```python
from build123d import *

# Parameters (mm, degrees)
SKETCH1_W                = 34
SKETCH1_H                = 24
BOSS_EXTRUDE1_DEPTH      = 10
SKETCH2_W                = 30
SKETCH2_H                = 20
CUT_EXTRUDE1_DEPTH       = 8
SKETCH3_W                = 16
SKETCH3_H                = 2
BOSS_EXTRUDE2_DEPTH      = 0.5
CHAMFER1_SIZE            = 0.5
SKETCH4_W                = 7
SKETCH4_H                = 7
BOSS_EXTRUDE3_DEPTH      = 3
FILLET1_R                = 3.5
SKETCH6_R                = 1.75
CUT_EXTRUDE2_DEPTH       = 29.635642127
CIRPATTERN2_COUNT        = 2
FILLET1_OF_CIRPATTERN2_R = 3.5
FILLET2_R                = 3.5


with BuildPart() as part:
    # Sketch1 → Boss-Extrude1 (new body)
    with BuildSketch(Plane.XY):
        Rectangle(SKETCH1_W, SKETCH1_H)
    extrude(amount=BOSS_EXTRUDE1_DEPTH)

    # Sketch2 → Cut-Extrude1 (cut)
    with BuildSketch(Plane.XY.offset(10)):
        Rectangle(SKETCH2_W, SKETCH2_H)
    extrude(amount=-CUT_EXTRUDE1_DEPTH, mode=Mode.SUBTRACT)

    # Sketch3 → Boss-Extrude2 (add)
    with BuildSketch(Plane.XZ.offset(-10)):
        with Locations((0, 9)):
            Rectangle(SKETCH3_W, SKETCH3_H)
    boss_extrude2 = extrude(amount=BOSS_EXTRUDE2_DEPTH)

    # Mirror1: Boss-Extrude2 across plane
    add(boss_extrude2.mirror(Plane.ZX))

    # Chamfer1
    chamfer1_edges = [part.edges().sort_by_distance(p)[0] for p in [
        (8, 10, 9),
        (-8, 10, 9),
        (-8, -10, 9),
        (8, -10, 9),
    ]]
    chamfer(chamfer1_edges, length=CHAMFER1_SIZE - 0.0001)  # a hair under: the kernel refuses the full size

    # Sketch4 → Boss-Extrude3 (add)
    with BuildSketch(Plane.XY):
        with Locations((20.5, 8.5)):
            Rectangle(SKETCH4_W, SKETCH4_H)
    boss_extrude3 = extrude(amount=BOSS_EXTRUDE3_DEPTH)

    # Fillet1
    fillet1_edges = [part.edges().sort_by_distance(p)[0] for p in [
        (24, 12, 1.5),
        (24, 5, 1.5),
    ]]
    fillet(fillet1_edges, radius=FILLET1_R - 0.0001)  # a hair under: the kernel refuses the full size

    # Sketch6 → Cut-Extrude2 (cut, through all)
    with BuildSketch(Plane(origin=(0, 0, 0), x_dir=(-1, 0, 0), z_dir=(0, 0, -1))):
        with Locations((-20.5, 8.5)):
            Circle(SKETCH6_R)
    cut_extrude2 = extrude(amount=-CUT_EXTRUDE2_DEPTH, mode=Mode.SUBTRACT)

    # CirPattern2: Boss-Extrude3, Cut-Extrude2 ×2 about axis
    cirpattern2_axis = Axis((0, 0, 0), (0, 0, 1))
    add([boss_extrude3.rotate(cirpattern2_axis, i * 360 / CIRPATTERN2_COUNT) for i in range(1, CIRPATTERN2_COUNT)])
    add([cut_extrude2.rotate(cirpattern2_axis, i * 360 / CIRPATTERN2_COUNT) for i in range(1, CIRPATTERN2_COUNT)], mode=Mode.SUBTRACT)

    # Fillet1 of CirPattern2
    fillet1_of_cirpattern2_edges = [part.edges().sort_by_distance(p)[0] for p in [
        (-24, -12, 1.5),
        (-24, -5, 1.5),
    ]]
    fillet(fillet1_of_cirpattern2_edges, radius=FILLET1_OF_CIRPATTERN2_R - 0.0001)  # a hair under: the kernel refuses the full size

    # Fillet2
    fillet2_edges = [part.edges().sort_by_distance(p)[0] for p in [
        (-17, -5, 1.5),
        (17, 5, 1.5),
    ]]
    fillet(fillet2_edges, radius=FILLET2_R)


solid = part.part
```
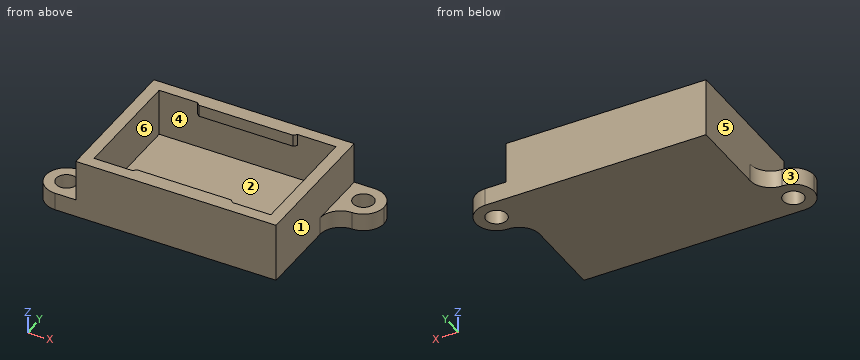
Design review of the part built by this model. Coordinates are the model's own, in mm. Face numbers are marked on the shaded views. A direction names the side the tool comes from. Round coordinates to 2 decimals unless told otherwise and drop trailing zeros. Order: outer loops, then holes, each group sorted by start corner. A loop starts at its lowest first (then second) coordinate and runs counter-clockwise, first axis right, second up. Notation, with made-up numbers: M 16.25,16 L 42.25,16 A15 cw 42.25,42 Z; hole C 23,-35.5 d11. An arc over 180 degrees is marked long. Put each result on its own line as item: value.
Q1. Insertion check: pin 1 Ø5 at (y, z) = (-3.5, 8.5) entering from +X; pin 2 Ø1 at (x, y) = (-3.5, 8.5) entering from +Z; pin 3 Ø3 at (y, z) = (3, 7) entering from -X. Each pin has a flat end and moves straight along its axis. Give the tip position at first contact, or say it passes through.
Reported:
pin 1: x = 17
pin 2: z = 2
pin 3: x = -17
Q2. Draft analysis for pull direction Y (two halves, no side actions). For the marked faces 1, 2 and 3, state which applies: released by +Y, released by -Y, zero draft, split by the parting line, or undercut.
Reported:
face 1: zero draft
face 2: undercut
face 3: released by +Y
Q3. Consider section B-B (z = 6). State the section outline as (x, y) points, and give its area (3 significant figures).
Reported:
outline: M -17,-12 L 17,-12 L 17,12 L -17,12 Z; hole M -15,-10 L 15,-10 L 15,10 L -15,10 Z
area: 216 mm²
Q4. Machinability: for the marked faces 4, 5 and 6, which of the approach directions +Z, -Z, +X, -X, +Y, -Y give a long, thin tool a straight path to every point of the face, cutting with its end or side? Answer none if there is none.
Reported:
face 4: none
face 5: +Z, -X, +Y
face 6: +Z
Q5. To check wall thickness, follow line 1 (Y direction, x = -20.5, z = 1.35); line 2 (Y direction, x = -4, z = 4.75); line 3 (X direction, y = -1.25, z = 3.5). State the ranges of each line that lie inside material, in increasing order.
Reported:
line 1: -12 to -10.25, -6.75 to -5
line 2: -12 to -10, 10 to 12
line 3: -17 to -15, 15 to 17
Q6. Consider section A-A (x = 1.5). State the section outline as (y, z) points.
Reported:
outline: M -12,0 L 12,0 L 12,10 L 9.5,10 L 9.5,8 L 10,8 L 10,2 L -10,2 L -10,8 L -9.5,8 L -9.5,10 L -12,10 Z
Q7. Consider section C-C (y = 2.25). State the section outline as (x, z) points.
Reported:
outline: M -17,0 L 17.08,0 L 17.08,3 L 17,3 L 17,10 L 15,10 L 15,2 L -15,2 L -15,10 L -17,10 Z
Q8. Consider section D-D (x = -20). State the section outline as (y, z) points.
Reported:
outline: M -12,0 L -10.18,0 L -10.18,3 L -12,3 Z; M -6.82,0 L -4.96,0 L -4.96,3 L -6.82,3 Z
